Autodesk Inventor part; units mm, degrees
ref_plane "Work Plane2" through (26.4443, -15.3077, 20) normal (1, 0, 0) x (0, 1, 0)
ref_plane "YZ Plane" through (0, 0, 0) normal (1, 0, 0) x (0, 1, 0)
ref_plane "XZ Plane" through (0, 0, 0) normal (0, 1, 0) x (-1, 0, 0)
sketch "Sketch1" plane through (0, 0, 0) normal (0, 0, 1) x (1, 0, 0)
  line L0 (-35, 19) -> (35, 19)
  line L1 (35, 19) -> (35, -19)
  line L2 (35, -19) -> (-35, -19)
  line L3 (-35, -19) -> (-35, 19)
  line L4 (-35, 19) -> (35, -19) construction
  line L5 (35, 19) -> (-35, -19) construction
  point P0 (0, 0)
  dimension "d0" = 70
  dimension "d1" = 38
extrude "Extrusion1" add sketch "Sketch1" along normal blind 20
sketch "Sketch2" plane through (0, 0, 20) normal (0, 0, 1) x (1, 0, 0)
  circle A0 centre (26.4443, -15.3077) radius 1.5
  circle A1 centre (30.4443, -15.3077) radius 1.5
  point P0 (0, 0)
  dimension "d4" = 3
  dimension "d5" = 3
  dimension "d6" = 4
ref_plane "Work Plane2" through (26.4443, -15.3077, 20) normal (1, 0, 0) x (0, 1, 0)
sketch "Sketch3" plane through (26.4443, -15.3077, 20) normal (1, 0, 0) x (0, 1, 0)
  line L0 (0, 0) -> (-8.28, 12.6748) construction
  line L1 (-8.28, 12.6748) -> (-23.4846, 12.6748) construction
  line L2 (-23.4846, 12.6748) -> (-18.7913, 40.4591) construction
  spline S0 degree 3 poles (0, 0) (-8.28, 12.6748) (-23.4846, 12.6748) (-18.7913, 40.4591) knots 1 1 1 1 2 2 2 2
  point P0 (15.3077, -20)
sweep "Sweep1" add profiles "Sketch2" path "Sketch3" contours A0
pattern_linear "Rectangular Pattern1" count 2 spacing 4 along (1, 0, 0) of "Sweep1"
properties part number "battery_5V"
For this review, take the finished solid that the model builds, in its own axes (mm). Coordinates: 2 decimals unless noted, no trailing zeros. Order: outer loops, then holes, each group sorted by start corner. A loop starts at its lowest first (then second) coordinate and runs counter-clockwise, first axis right, second up. Notation, with made-up numbers: (80, 7.5) -> (103, 7.5) arc R3 cw to (103, 12.5) -> close; hole circle Ø2 at (22, -27.75). An arc over 180 degrees is marked (long way). Return JSON: item names as keys, results as strings.
1. We need section B-B on z = 4. Write out the cut boundary in (x, y).
Answer block:
{"outline": "(-35, -19) -> (35, -19) -> (35, 19) -> (-35, 19) -> close"}
2. For line 1 (Z direction, x = -3, y = 17); line 2 (Y direction, x = 22.5, z = 8.5), list the stretches that pass through material, from the lowest coordinate up. Write a range as from..to.
Answer block:
{"line 1": "0..20", "line 2": "-19..19"}
3. We need section A-A on y = 9.5. Write out the cut boundary in (x, z).
Answer block:
{"outline": "(-35, 0) -> (35, 0) -> (35, 20) -> (-35, 20) -> close"}
4. For pin 1 Ø16 at (x, z) = (3.5, 14) entering from -Y; pin 2 Ø5 at (x, y) = (14, -1) entering from +Z, all flat-tipped, find the tip position at first contact; note any pin that passes through.
Answer block:
{"pin 1": "y = -19", "pin 2": "z = 20"}
